Part model, mm, in its own coordinate system. Round coordinates to 2 decimals unless told otherwise and drop trailing zeros. Loops run counter-clockwise (first coordinate to the right, second up) from the corner with the lowest first, then second, coordinate; pieces in that order, holes last. Notation, with made-up numbers: (86.5, -19.5) -> (90.5, -19.5) arc R17 ccw to (90.5, -5.5) -> close; hole circle Ø4 at (-24.75, 76.25). An arc over 180 degrees is marked (long way). Answer as CSV lines item,"result".
from build123d import *

# Parameters (mm, degrees)
ESQUISSE1_R             = 6
ESQUISSE1_R_2           = 3
BOSS_EXTRU_1_DEPTH      = 2
CONG_1_R                = 18
CONG_2_R                = 20
D_GAGEMENT_M32_D        = 3.4
ENL_V_MAT_EXTRU_1_DEPTH = 234.819122898
ENL_V_MAT_EXTRU_2_DEPTH = 234.819122898
ESQUISSE8_R             = 1.6
ENL_V_MAT_EXTRU_3_DEPTH = 234.819122898
D_GAGEMENT_M51_D        = 5.5
D_GAGEMENT_M52_D        = 5.5
ESQUISSE13_W            = 20
ESQUISSE13_H            = 20
ENL_V_MAT_EXTRU_4_DEPTH = 234.819122898
CONG_3_R                = 2


with BuildPart() as part:
    # Esquisse1 → Boss.-Extru.1 (new body)
    with BuildSketch(Plane.XY):
        Polygon((-284.958991582, 40), (-247.300009613, 40), (248.333273954, 40), (284.958991582, 40), (248.333273954, 20.647569508), (152.479495791, -30), (-152.479495791, -30), (-247.300009613, 20.10160952), align=None)
        with Locations((-215, 20)):
            Circle(ESQUISSE1_R, mode=Mode.SUBTRACT)
        with Locations((-150, -20)):
            Circle(ESQUISSE1_R_2, mode=Mode.SUBTRACT)
        with Locations((150, -20)):
            Circle(ESQUISSE1_R_2, mode=Mode.SUBTRACT)
        with Locations((215, 20)):
            Circle(ESQUISSE1_R_2, mode=Mode.SUBTRACT)
        with Locations((0, -20)):
            Circle(ESQUISSE1_R_2, mode=Mode.SUBTRACT)
        with Locations((-71.666666667, 20)):
            Circle(ESQUISSE1_R, mode=Mode.SUBTRACT)
        with Locations((71.666666667, 20)):
            Circle(ESQUISSE1_R_2, mode=Mode.SUBTRACT)
    extrude(amount=BOSS_EXTRU_1_DEPTH)

    # Congé1
    cong_1_edges = [part.edges().sort_by_distance(p)[0] for p in [
        (-284.958991582, 40, 1),
        (284.958991582, 40, 1),
    ]]
    fillet(cong_1_edges, radius=CONG_1_R)

    # Congé2
    cong_2_edges = [part.edges().sort_by_distance(p)[0] for p in [
        (152.479495791, -30, 1),
        (-152.479495791, -30, 1),
    ]]
    fillet(cong_2_edges, radius=CONG_2_R)

    # Dégagement M32 (through all)
    with Locations(Plane(origin=(0, 0, 0), x_dir=(-1, 0, 0), z_dir=(0, 0, -1))):
        with Locations((-200, 33.228756555), (-200, 6.771243445)):
            Hole(D_GAGEMENT_M32_D / 2)

    # Esquisse4 → Enlèv. mat.-Extru.1 (cut, through all)
    with BuildSketch(Plane(origin=(0, 0, 0), x_dir=(-1, 0, 0), z_dir=(0, 0, -1))):
        with BuildLine():
            Line((-229.334149786, 16), (-205, 16))
            ThreePointArc((-205, 16), (-201, 20), (-205, 24))
            Line((-205, 24), (-230.252130857, 24))
            ThreePointArc((-230.252130857, 24), (-230.246241418, 19.948007721), (-229.334149786, 16))
        make_face()
    extrude(amount=-ENL_V_MAT_EXTRU_1_DEPTH, mode=Mode.SUBTRACT)

    # Esquisse7 → Enlèv. mat.-Extru.2 (cut, through all)
    with BuildSketch(Plane(origin=(0, 0, 0), x_dir=(-1, 0, 0), z_dir=(0, 0, -1))):
        with BuildLine():
            ThreePointArc((-200, 5.071243445), (-201.7, 6.771243445), (-200, 8.471243445))
            Line((-200, 8.471243445), (-210, 8.471243445))
            ThreePointArc((-210, 8.471243445), (-211.7, 6.771243445), (-210, 5.071243445))
            Line((-210, 5.071243445), (-200, 5.071243445))
        make_face()
        with BuildLine():
            Line((-190, 8.471243445), (-200, 8.471243445))
            ThreePointArc((-200, 8.471243445), (-198.797918472, 7.973324973), (-198.3, 6.771243445))
            ThreePointArc((-198.3, 6.771243445), (-198.797918472, 5.569161917), (-200, 5.071243445))
            Line((-200, 5.071243445), (-190, 5.071243445))
            ThreePointArc((-190, 5.071243445), (-188.3, 6.771243445), (-190, 8.471243445))
        make_face()
        with BuildLine():
            Line((-190, 34.928756555), (-200, 34.928756555))
            ThreePointArc((-200, 34.928756555), (-198.797918472, 34.430838083), (-198.3, 33.228756555))
            ThreePointArc((-198.3, 33.228756555), (-198.797918472, 32.026675027), (-200, 31.528756555))
            Line((-200, 31.528756555), (-190, 31.528756555))
            ThreePointArc((-190, 31.528756555), (-188.3, 33.228756555), (-190, 34.928756555))
        make_face()
        with BuildLine():
            ThreePointArc((-200, 31.528756555), (-201.7, 33.228756555), (-200, 34.928756555))
            Line((-200, 34.928756555), (-210, 34.928756555))
            ThreePointArc((-210, 34.928756555), (-211.7, 33.228756555), (-210, 31.528756555))
            Line((-210, 31.528756555), (-200, 31.528756555))
        make_face()
    extrude(amount=-ENL_V_MAT_EXTRU_2_DEPTH, mode=Mode.SUBTRACT)

    # Esquisse8 → Enlèv. mat.-Extru.3 (cut, through all)
    with BuildSketch(Plane(origin=(0, 0, 0), x_dir=(-1, 0, 0), z_dir=(0, 0, -1))):
        with Locations((221.423393759, 27.75)):
            Circle(ESQUISSE8_R)
        with Locations((208, 35.5)):
            Circle(ESQUISSE8_R)
        with Locations((194.576606241, 27.75)):
            Circle(ESQUISSE8_R)
        with Locations((194.576606241, 12.25)):
            Circle(ESQUISSE8_R)
        with Locations((208, 4.5)):
            Circle(ESQUISSE8_R)
        with Locations((221.423393759, 12.25)):
            Circle(ESQUISSE8_R)
        with Locations((78.090060425, 27.75)):
            Circle(ESQUISSE8_R)
        with Locations((64.666666667, 35.5)):
            Circle(ESQUISSE8_R)
        with Locations((51.243272908, 27.75)):
            Circle(ESQUISSE8_R)
        with Locations((51.243272908, 12.25)):
            Circle(ESQUISSE8_R)
        with Locations((64.666666667, 4.5)):
            Circle(ESQUISSE8_R)
        with Locations((78.090060425, 12.25)):
            Circle(ESQUISSE8_R)
    extrude(amount=-ENL_V_MAT_EXTRU_3_DEPTH, mode=Mode.SUBTRACT)

    # Dégagement M51 (through all)
    with Locations(Plane(origin=(0, 0, 0), x_dir=(-1, 0, 0), z_dir=(0, 0, -1))):
        with Locations((143.333333333, 20), (0, 20), (-143.333333333, 20)):
            Hole(D_GAGEMENT_M51_D / 2)

    # Dégagement M52 (through all)
    with Locations(Plane.XY.offset(2)):
        with Locations((-75, -20), (75, -20)):
            Hole(D_GAGEMENT_M52_D / 2)

    # Esquisse13 → Enlèv. mat.-Extru.4 (cut, through all)
    with BuildSketch(Plane.XY.offset(2)):
        with Locations((-143.333333333, 20)):
            Rectangle(ESQUISSE13_W, ESQUISSE13_H)
        with Locations((0, 20)):
            Rectangle(ESQUISSE13_W, ESQUISSE13_H)
    extrude(amount=-ENL_V_MAT_EXTRU_4_DEPTH, mode=Mode.SUBTRACT)

    # Congé3
    cong_3_edges = [part.edges().sort_by_distance(p)[0] for p in [
        (-133.333333333, 30, 1),
        (-133.333333333, 10, 1),
        (-153.333333333, 10, 1),
        (-153.333333333, 30, 1),
        (10, 30, 1),
        (10, 10, 1),
        (-10, 10, 1),
        (-10, 30, 1),
    ]]
    fillet(cong_3_edges, radius=CONG_3_R)


solid = part.part
Q1. Saw through at A-A, the plane z = 0.8. Give the number of separate pieces and of enclosed holes in the cut face, then the cut area to 3 significant figures.
Geometry results:
separate pieces,"1"
enclosed holes,"25"
area,"27,200 mm2"
Q2. Drill centre lines: line 1 along Y through (x, z) = (75, 0.9); line 2 along Y through (x, z) = (-2, 1.8); line 3 along Y through (x, z) = (-5.5, 0.3). Where is each one in solid material? Low to high.
Geometry results:
line 1,"-30 to -22.75, -17.25 to 40"
line 2,"-30 to -22.24, -17.76 to 10, 30 to 40"
line 3,"-30 to 10, 30 to 40"
Q3. Drop flat-ended pins along their axis: P1, Ø5, axis at x = -75, y = -20, coming from the +Z side; P2, Ø3.5, axis at x = -221.42, y = 12.25, coming from the +Z side; P3, Ø1, axis at x = 217, z = 1, coming from the +Y side; P4, Ø1, axis at x = 203, z = 1.5, coming from the -Y side. Give the stop position or say it passes through.
Geometry results:
P1,"through"
P2,"z = 2"
P3,"y = 39.52"
P4,"y = -3.57"
Q4. Two-plate mould, pull along X, no slides. Class faces 1 (the face through (3, 5, 2)), 2 (the face through (-219.76, 16.35, 0.99)), 3 (the face through (189.27, -10.56, 0.99)): pulls with the +X half, pulls with the -X half, needs draft (parallel to the pull), parting line crosses it, or undercut.
Geometry results:
face 1,"needs draft"
face 2,"undercut"
face 3,"pulls with the +X half"
Q5. Saw through at B-B, the plane y = -2. Write the cut outline in (x, z).
Geometry results:
outline,"(-205.47, 0) -> (205.47, 0) -> (205.47, 2) -> (-205.47, 2) -> close"
